For this review, take the finished solid that the model builds, in its own axes (mm). A direction names the side the tool comes from. Coordinates: 2 decimals unless noted, no trailing zeros. Loops run counter-clockwise (first coordinate to the right, second up) from the corner with the lowest first, then second, coordinate; pieces in that order, holes last. Notation, with made-up numbers: (2, 67.25) -> (33, 67.25) arc R6 ccw to (33, 72.25) -> close; hole circle Ø2 at (-4.75, 86.5). An arc over 180 degrees is marked (long way). Answer in a Markdown table with one row per item.
from build123d import *

# Parameters (mm, degrees)
SKETCH1_W           = 10
SKETCH1_H           = 25
BOSS_EXTRUDE1_DEPTH = 3
SKETCH3_W           = 3
SKETCH3_H           = 7
BOSS_EXTRUDE2_DEPTH = 10
BOSS_EXTRUDE3_DEPTH = 20
BOSS_EXTRUDE4_DEPTH = 10


with BuildPart() as part:
    # Sketch1 → Boss-Extrude1 (new body)
    with BuildSketch(Plane.XY):
        with Locations((0, 22.5)):
            Rectangle(SKETCH1_W, SKETCH1_H)
        with BuildLine():
            ThreePointArc((-1.6, 31.6), (0, 33.2), (1.6, 31.6))
            Line((1.6, 31.6), (1.6, 21.6))
            ThreePointArc((1.6, 21.6), (0, 20), (-1.6, 21.6))
            Line((-1.6, 21.6), (-1.6, 31.6))
        make_face(mode=Mode.SUBTRACT)
    extrude(amount=BOSS_EXTRUDE1_DEPTH)

    # Sketch3 → Boss-Extrude2 (add)
    with BuildSketch(Plane(origin=(5, 0, 0), x_dir=(0, 0, -1), z_dir=(1, 0, 0))):
        Polygon((0, 7), (0, 10), (-3, 10), (-7, 10), (-7, 7), (-4, 7), align=None)
        with Locations((-5.5, 3.5)):
            Rectangle(SKETCH3_W, SKETCH3_H)
    extrude(amount=-BOSS_EXTRUDE2_DEPTH)

    # Sketch4 → Boss-Extrude3 (add)
    with BuildSketch(Plane(origin=(5, 0, 0), x_dir=(0, 0, -1), z_dir=(1, 0, 0))):
        Polygon((-19, -9.660254038), (-4, 0), (-7, 0), (-19, 0), align=None)
        Polygon((-4, -1), (-19, -9.660254038), (-4, 0), align=None)
    extrude(amount=-BOSS_EXTRUDE3_DEPTH)

    # Sketch5 → Boss-Extrude4 (add)
    with BuildSketch(Plane.ZY.offset(5)):
        Polygon((4, 7), (0, 7), (4, 0), align=None)
        Polygon((3, 18), (0, 7), (4, 7), (4, 0), (19, 0), (9.027600975, 11.218948904), align=None)
    extrude(amount=-BOSS_EXTRUDE4_DEPTH)


solid = part.part
Item 1: Insertion check: pin 1 (8 mm diameter, centred on x = -1.5, y = 26.5, fed in from +Z); pin 2 (1.5 mm diameter, centred on x = -5.5, z = 14, fed in from -Y); pin 3 (2.5 mm diameter, centred on y = 29, z = 1.5, fed in from -X). Each pin has a flat end and moves straight along its axis. Give the tip position at first contact, or say it passes through.
Worked answers:
| item | result |
|---|---|
| pin 1 | z = 3 |
| pin 2 | y = -7.21 |
| pin 3 | x = -5 |
Item 2: The part is to be moulded in two halves that separate along X. For faces 1 (the flat face through (5, 8, 7)), 2 (the flat face through (-5, 12, 6)), 3 (the cylindrical face through (0, 20, 1)), say which applies: +X half, -X half, draft (parallel to the pull), parting line (faces both ways), or undercut.
Worked answers:
| item | result |
|---|---|
| face 1 | +X half |
| face 2 | -X half |
| face 3 | undercut |
Item 3: Take a section at A-A, the plane x = 0. State the section outline as (y, z) points, and give its area (3 significant figures).
Worked answers:
| item | result |
|---|---|
| outline | (-9.66, 19) -> (-1, 4) -> (0, 4) -> (7, 0) -> (20, 0) -> (20, 3) -> (18, 3) -> (0, 19) -> close; (33.2, 0) -> (35, 0) -> (35, 3) -> (33.2, 3) -> close |
| area | 275 mm² |
Item 4: Take a section at C-C, the plane z = 5.25. State the section outline as (x, y) points.
Worked answers:
| item | result |
|---|---|
| outline | (-15, -1.72) -> (5, -1.72) -> (5, 15.47) -> (-5, 15.47) -> (-5, 0) -> (-15, 0) -> close |
Item 5: Take a section at D-D, the plane x = -12.25. State the section outline as (y, z) points.
Worked answers:
| item | result |
|---|---|
| outline | (-9.66, 19) -> (-1, 4) -> (0, 4) -> (0, 19) -> close |
Item 6: Take a section at B-B, the plane z = 2.5. State the section outline as (x, y) points (3 decimals), and give its area (3 significant figures).
Worked answers:
| item | result |
|---|---|
| outline | (-5, 2.625) -> (5, 2.625) -> (5, 35) -> (-5, 35) -> close; hole (-1.6, 21.6) arc R1.6 ccw to (1.6, 21.6) -> (1.6, 31.6) arc R1.6 ccw to (-1.6, 31.6) -> close |
| area | 284 mm² |
Item 7: For faces 4 (the flat face through (-4.9, -0.5, 4)), 5 (the flat face through (1.6, 27, 1)), 6 (the flat face through (-2, 27, 3)), 7 (the flat face through (-5, -5, 19)), 8 (the flat face through (-10, 0, 11)), list the 3-axis set-ups (+Z, -Z, +X, -X, +Y, -Y) from which the entire face can be reached by the end or side of a thin tool; tool diameter is ignored.
Worked answers:
| item | result |
|---|---|
| face 4 | -Z, +X, -X, -Y |
| face 5 | +Z, -Z |
| face 6 | +Z, +X, -X, +Y |
| face 7 | +Z, +X, -X, +Y, -Y |
| face 8 | +Z, -Z, -X, +Y |
Item 8: For L1, parallel to X at y = 14.5, z = 4.5; L2, parallel to Z at x = 0, y = 8.5; L3, parallel to Y at x = -8.25, z = 9, list the stretches that pass through material, from the lowest coordinate up.
Worked answers:
| item | result |
|---|---|
| L1 | -5 to 5 |
| L2 | 0 to 11.44 |
| L3 | -3.89 to 0 |
